The listing builds one solid part. Answer for the finished solid, in the listing's coordinates (mm). Face numbers are marked on the shaded views. Coordinates: 2 decimals unless noted, no trailing zeros. Loops run counter-clockwise (first coordinate to the right, second up) from the corner with the lowest first, then second, coordinate; pieces in that order, holes last. Notation, with made-up numbers: (-29, -15) - (-20, -15) arc R31 cw to (-20, 15) - close; hole circle Ø8 at (-24, 37). An arc over 180 degrees is marked (long way). Return JSON: item names as keys, results as strings. Group by question number.
1. Section D-D (z = 12.5) is taken. Write down the section's boundary in (x, y), and give its area (3 significant figures).
2. Each of these flat-tipped pins is pushed along its axis until it touches: P1, Ø6, axis at x = -43, z = 43.5, coming from the -Y side; P2, Ø12, axis at y = -6.5, z = 29, coming from the -X side; P3, Ø1.5, axis at y = -34, z = 38, coming from the -X side. Where does it stop, or does it pass through?
3. Section A-A (z = 48) is taken. Write down the section's boundary in (x, y), and give its area (3 significant figures).
4. Find the intervals of material crossed by line 1 along Y through (x, z) = (7, 48.5); line 2 along X through (y, z) = (-61, 44); line 3 along X through (y, z) = (-16, 8.5), in increasing order.
5. The mould has two halves that part along Y. Classify the marked faces 1, 2, 3 and 4: pulls with the +Y half, pulls with the -Y half, needs draft (parallel to the pull), parting line crosses it, or undercut.
6. Section C-C (y = -55.5) is taken. Write down the section's boundary in (x, z).
7. Section B-B (x = -54.5) is taken. Write down the section's boundary in (y, z), and give its area (3 significant figures).
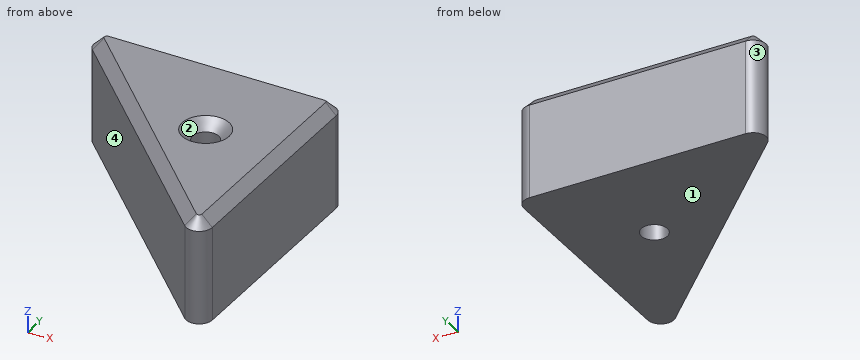
```python
from build123d import *

# Parameters (mm, degrees)
F1_DEPTH = 50.8
F2_SIZE  = 5.08


with BuildPart() as f1:
    # F0 (on Top) → F1 (new body)
    with BuildSketch(Plane.XY):
        with BuildLine():
            Line((38.243972, 34.775752), (-67.075772, 34.775752))
            ThreePointArc((-67.075772, 34.775752), (-72.942407, 30.855792), (-71.5659, 23.935624))
            Line((-71.5659, 23.935624), (33.753843, -81.38412))
            ThreePointArc((33.753843, -81.38412), (40.674011, -82.760627), (44.593972, -76.893992))
            Line((44.593972, -76.893992), (44.593972, 28.425752))
            ThreePointArc((44.593972, 28.425752), (42.7341, 32.91588), (38.243972, 34.775752))
        make_face()
        with BuildLine():
            ThreePointArc((0.143972, -16.024248), (6.493972, -9.674248), (12.843972, -16.024248))
            ThreePointArc((12.843972, -16.024248), (6.493972, -22.374248), (0.143972, -16.024248))
        make_face(mode=Mode.SUBTRACT)
    extrude(amount=F1_DEPTH)

    # F2
    f2_edges = [f1.edges().sort_by_distance(p)[0] for p in [
        (44.593972, -24.23412, 50.8),
        (0.143972, -16.024248, 50.8),
    ]]
    chamfer(f2_edges, length=F2_SIZE)


solid = f1.part
```
The answers:
{
 "1": {"outline": "(-71.57, 23.94) - (33.75, -81.38) arc R6.35 ccw to (44.59, -76.89) - (44.59, 28.43) arc R6.35 ccw to (38.24, 34.78) - (-67.08, 34.78) arc R6.35 ccw to start; hole circle Ø12.7 at (6.49, -16.02)", "area": "7,830 mm2"},
 "2": {"P1": "stops at y = -7.63", "P2": "stops at x = -47.13", "P3": "stops at x = -14.38"},
 "3": {"outline": "(-69.95, 25.55) - (35.37, -79.77) arc R4.07 ccw to (42.31, -76.89) - (42.31, 28.43) arc R4.07 ccw to (38.24, 32.5) - (-67.08, 32.5) arc R4.07 ccw to start; hole circle Ø17.26 at (6.49, -16.02)", "area": "6,830 mm2"},
 "4": {"line 1": "y = -50.7 to -25.14, -6.91 to 32", "line 2": "x = 13.37 to 44.59", "line 3": "x = -31.63 to 0.14, 12.84 to 44.59"},
 "5": {"face 1": "needs draft", "face 2": "undercut", "face 3": "parting line crosses it", "face 4": "pulls with the -Y half"},
 "6": {"outline": "(7.87, 0) - (44.59, 0) - (44.59, 45.72) - (39.51, 50.8) - (15.05, 50.8) - (7.87, 45.72) - close"},
 "7": {"outline": "(6.87, 0) - (34.78, 0) - (34.78, 45.72) - (29.7, 50.8) - (14.05, 50.8) - (6.87, 45.72) - close", "area": "1,390 mm2"}
}
